```python
from build123d import *

# Parameters (mm, degrees)
FILLET1_R                = 0.1
SKETCH3_W                = 0.48
SKETCH3_H                = 2.1
SKETCH4_W                = 0.48
SKETCH4_H                = 0.68402847
RECPAT_COUNT             = 2
RECPAT_ANGLE             = 90
THDSCHPAT_COUNT          = 11
THDSCHPAT_PITCH          = 0.4
ESBO_O1_R                = 2.4
RESSALTO_EXTRUS_O1_DEPTH = 0.5


with BuildPart() as part:
    # BodySke → Base-Revolve (revolve)
    with BuildSketch(Plane.XY):
        with BuildLine():
            Line((1.6, 1), (1.6, 2))
            Line((1.6, 2), (1.1, 2))
            ThreePointArc((1.1, 2), (0.688403396, 1.885994341), (0.394117647, 1.576470588))
            ThreePointArc((0.394117647, 1.576470588), (0.100022625, 0.812494344), (0, 0))
            Line((0, 0), (23.6, 0))
            Line((23.6, 0), (23.6, 1))
            Line((23.6, 1), (1.6, 1))
        make_face()
    revolve(axis=Axis((-25.4, 0, 0), (1, 0, 0)))

    # Fillet1
    fillet1_edges = [part.edges().sort_by_distance(p)[0] for p in [
        (1.6, -1, 0),
    ]]
    fillet(fillet1_edges, radius=FILLET1_R)

    # Sketch3 → Recess section 0
    with BuildSketch(Plane(origin=(0, 0, 0), x_dir=(0, 0, -1), z_dir=(1, 0, 0))):
        Rectangle(SKETCH3_W, SKETCH3_H)
    # Sketch4 → Recess section 1
    with BuildSketch(Plane(origin=(1.42, 0, 0), x_dir=(0, 0, -1), z_dir=(1, 0, 0))):
        Rectangle(SKETCH4_W, SKETCH4_H)
    recess = loft(mode=Mode.SUBTRACT)

    # RecPat: Recess ×2 about axis
    recpat_axis = Axis((0, 0, 0), (1, 0, 0))
    for i in range(1, RECPAT_COUNT):
        add(recess.rotate(recpat_axis, i * RECPAT_ANGLE / (RECPAT_COUNT - 1)), mode=Mode.SUBTRACT)

    # RecCorSke → RecessCore (revolve, cut)
    with BuildSketch(Plane.XY):
        Polygon((0, 0), (0, 0.454796073), (1.42, 0.3555), (1.535508952, 0), align=None)
    revolve(axis=Axis((-3.175, 0, 0), (1, 0, 0)), mode=Mode.SUBTRACT)

    # ThdSchSke → ThreadSchematic (revolve, cut)
    with BuildSketch(Plane.XY):
        Polygon((19.6, -0.774), (19.441753096, -1), (19.441753096, -1.25), (19.758246904, -1.25), (19.758246904, -1), align=None)
    threadschematic = revolve(axis=Axis((-3.175, 0, 0), (1, 0, 0)), mode=Mode.SUBTRACT)

    # ThdSchPat: ThreadSchematic ×11
    with Locations(*[(i * THDSCHPAT_PITCH, 0, 0) for i in range(1, THDSCHPAT_COUNT)]):
        add(threadschematic, mode=Mode.SUBTRACT)

    # Esboço1 → Ressalto-extrusão1 (add)
    with BuildSketch(Plane(origin=(1.6, 0, 0), x_dir=(0, 0, -1), z_dir=(1, 0, 0))):
        Circle(ESBO_O1_R)
    extrude(amount=-RESSALTO_EXTRUS_O1_DEPTH)


solid = part.part
```
Could you check a few things on this model? Use its own coordinates, in mm. Round coordinates to 2 decimals unless told otherwise and drop trailing zeros. Write each loop counter-clockwise with the first axis right and the second up, starting at its lowest first coordinate (ties: lowest second). Pieces come first, ordered by that corner, then holes.
(1) For pin 1 (2 mm diameter, centred on x = 5, z = 0.5, fed in from -Y), with a flat end and sliding along its axis, tell me the tip position at first contact or that it passes through.
Findings below:
pin 1: stops at y = -1
(2) If I drill on probe 1 along Z at (x, y) = (2, -0.2); probe 2 along X at (y, z) = (-0.45, -0.1); probe 3 along Y at (x, z) = (14.25, -0.1), over which ranges is the centre line in solid material (lowest first)?
Findings below:
probe 1: z = -0.98 to 0.98
probe 2: x = 1.1 to 23.6
probe 3: y = -0.99 to 0.99
(3) Suppose I cut it at A-A on x = 13.75. Write out the boundary of the cut face in (y, z), and give its area (3 significant figures).
Findings below:
outline: circle Ø2 at (0, 0)
area: 3.14 mm2
